Part model, mm, in its own coordinate system. A direction names the side the tool comes from. Round coordinates to 2 decimals unless told otherwise and drop trailing zeros. Write each loop counter-clockwise with the first axis right and the second up, starting at its lowest first coordinate (ties: lowest second). Pieces come first, ordered by that corner, then holes.
1) Saw through at B-B on z = 1.55. Write the cut outline in (x, y), and give its area (3 significant figures).
2) Which spindle directions (+Z, -Z, +X, -X, +Y, -Y) get a long thin tool onto all of the face, cutting with end or side? Do faces 1 (the flat face through (0, 12.5, 2)), 2 (the cylindrical face through (-12.15, 3.18, 1.27)), 3 (the flat face through (0, 9.5, 3)). Say none if no direction does.
3) Flat gauge pin, fed straight in: pin 1 (3 mm diameter, centred on x = 15, y = -6.75, fed in from +Z). Where does the tip first touch, or does it go through?
4) Saw through at D-D on y = -6.75. Write the cut outline in (x, z).
5) Saw through at C-C on x = 0. Write the cut outline in (y, z), and give its area (3 significant figures).
6) Saw through at A-A on x = 10. Write the cut outline in (y, z).
7) Pull direction X, two halves, no side cores. Call faces 4 (the flat face through (22.5, 0, 2)), 5 (the flat face through (0, -12.5, 2)), 6 (the flat face through (0, 4, 2.5)): +X half, -X half, draft (parallel to the pull), parting line (faces both ways), or undercut.
8) Drill centre lines: L1, parallel to Y at x = 0, z = 1.5; L2, parallel to Y at x = 10, z = 0.55; L3, parallel to Y at x = -8, z = 3.3. Where is each one in solid material? Low to high.
```python
from build123d import *

# Parameters (mm, degrees)
SKETCH1_W             = 45
SKETCH1_H             = 25
BOSS_EXTRUDE1_DEPTH   = 4
SKETCH2_W             = 37
SKETCH2_H             = 19
CUT_EXTRUDE1_DEPTH    = 1.5
FILLET1_R             = 2
CUT_EXTRUDE2_DEPTH    = 26.860201082
F_2_5MM_DOWEL_HOLE1_D = 2.5


with BuildPart() as part:
    # Sketch1 → Boss-Extrude1 (new body)
    with BuildSketch(Plane.XY):
        Rectangle(SKETCH1_W, SKETCH1_H)
    extrude(amount=BOSS_EXTRUDE1_DEPTH)

    # Sketch2 → Cut-Extrude1 (cut)
    with BuildSketch(Plane.XY.offset(4)):
        Rectangle(SKETCH2_W, SKETCH2_H)
    extrude(amount=-CUT_EXTRUDE1_DEPTH, mode=Mode.SUBTRACT)

    # Fillet1
    fillet1_edges = [part.edges().sort_by_distance(p)[0] for p in [
        (18.5, 9.5, 3.25),
        (18.5, -9.5, 3.25),
        (-18.5, -9.5, 3.25),
        (-18.5, 9.5, 3.25),
    ]]
    fillet(fillet1_edges, radius=FILLET1_R)

    # Sketch3 → Cut-Extrude2 (cut, through all)
    with BuildSketch(Plane.XY.offset(2.5)):
        with BuildLine():
            Line((-10.75, -3.75), (10.75, -3.75))
            ThreePointArc((10.75, -3.75), (12.164213562, -3.164213562), (12.75, -1.75))
            Line((12.75, -1.75), (12.75, 1.75))
            ThreePointArc((12.75, 1.75), (12.164213562, 3.164213562), (10.75, 3.75))
            Line((10.75, 3.75), (-10.75, 3.75))
            ThreePointArc((-10.75, 3.75), (-12.164213562, 3.164213562), (-12.75, 1.75))
            Line((-12.75, 1.75), (-12.75, -1.75))
            ThreePointArc((-12.75, -1.75), (-12.164213562, -3.164213562), (-10.75, -3.75))
        make_face()
    extrude(amount=-CUT_EXTRUDE2_DEPTH, mode=Mode.SUBTRACT)

    # Ø2.5mm Dowel Hole1 (through all)
    with Locations(Plane.XY.offset(2.5)):
        with Locations((-15, -6.75), (0, -6.75), (15, -6.75)):
            Hole(F_2_5MM_DOWEL_HOLE1_D / 2)


solid = part.part
```
Completed:
1. outline: (-22.5, -12.5) - (22.5, -12.5) - (22.5, 12.5) - (-22.5, 12.5) - close; hole circle Ø2.5 at (-15, -6.75); hole (-12.75, -1.75) arc R2 ccw to (-10.75, -3.75) - (10.75, -3.75) arc R2 ccw to (12.75, -1.75) - (12.75, 1.75) arc R2 ccw to (10.75, 3.75) - (-10.75, 3.75) arc R2 ccw to (-12.75, 1.75) - close; hole circle Ø2.5 at (0, -6.75); hole circle Ø2.5 at (15, -6.75)
1. area: 922 mm2
2. face 1: +Z, -Z, +X, -X, +Y
2. face 2: +Z, -Z
2. face 3: +Z
3. pin 1: stops at z = 2.5
4. outline: (-22.5, 0) - (-16.25, 0) - (-16.25, 2.5) - (-18.5, 2.5) - (-18.5, 4) - (-22.5, 4) - close; (-13.75, 0) - (-1.25, 0) - (-1.25, 2.5) - (-13.75, 2.5) - close; (1.25, 0) - (13.75, 0) - (13.75, 2.5) - (1.25, 2.5) - close; (16.25, 0) - (22.5, 0) - (22.5, 4) - (18.5, 4) - (18.5, 2.5) - (16.25, 2.5) - close
5. outline: (-12.5, 0) - (-8, 0) - (-8, 2.5) - (-9.5, 2.5) - (-9.5, 4) - (-12.5, 4) - close; (-5.5, 0) - (-3.75, 0) - (-3.75, 2.5) - (-5.5, 2.5) - close; (3.75, 0) - (12.5, 0) - (12.5, 4) - (9.5, 4) - (9.5, 2.5) - (3.75, 2.5) - close
5. area: 46.5 mm2
6. outline: (-12.5, 0) - (-3.75, 0) - (-3.75, 2.5) - (-9.5, 2.5) - (-9.5, 4) - (-12.5, 4) - close; (3.75, 0) - (12.5, 0) - (12.5, 4) - (9.5, 4) - (9.5, 2.5) - (3.75, 2.5) - close
7. face 4: +X half
7. face 5: draft
7. face 6: undercut
8. L1: y = -12.5 to -8, -5.5 to -3.75, 3.75 to 12.5
8. L2: y = -12.5 to -3.75, 3.75 to 12.5
8. L3: y = -12.5 to -9.5, 9.5 to 12.5
